from build123d import *

# Parameters (mm, degrees)
SKETCH1_R           = 24
SKETCH1_R_2         = 2
SKETCH1_R_3         = 1.5
BOSS_EXTRUDE1_DEPTH = 2
CUT_EXTRUDE1_DEPTH  = 2
FILLET1_R           = 1.5
SKETCH3_R           = 1.75
CUT_EXTRUDE2_DEPTH  = 10
SCALE1_SCALE        = 2
SKETCH4_R           = 5
CUT_EXTRUDE3_DEPTH  = 10
SKETCH5_R           = 6.547213639
SKETCH5_R_2         = 2.5
SKETCH5_R_3         = 5.064875416
BOSS_EXTRUDE2_DEPTH = 4


with BuildPart() as part:
    # Sketch1 → Boss-Extrude1 (new body)
    with BuildSketch(Plane(origin=(0, 0, 0), x_dir=(1, 0, 0), z_dir=(0, 1, 0))):
        with Locations(Location((0, 0, 0), (0, 0, 270))):
            Circle(SKETCH1_R)
        with Locations(Location((0, 0, 0), (0, 0, 270))):
            Circle(SKETCH1_R_2, mode=Mode.SUBTRACT)
        with Locations(Location((11.5, 0, 0), (0, 0, 270))):
            Circle(SKETCH1_R_3, mode=Mode.SUBTRACT)
        with Locations(Location((-5.75, -9.959292144, 0), (0, 0, 270))):
            Circle(SKETCH1_R_3, mode=Mode.SUBTRACT)
        with Locations(Location((-5.75, 9.959292144, 0), (0, 0, 270))):
            Circle(SKETCH1_R_3, mode=Mode.SUBTRACT)
    extrude(amount=BOSS_EXTRUDE1_DEPTH)

    # Sketch2 → Cut-Extrude1 (cut)
    with BuildSketch(Plane(origin=(0, 2, 0), x_dir=(1, 0, 0), z_dir=(0, 1, 0))):
        with BuildLine():
            Line((21.972994789, 3.5), (14.585952146, 3.5))
            ThreePointArc((14.585952146, 3.5), (7.5, 12.990381057), (-4.26188716, 14.381805097))
            Line((-4.26188716, 14.381805097), (-7.955408481, 20.779171685))
            ThreePointArc((-7.955408481, 20.779171685), (11.125, 19.269065234), (21.972994789, 3.5))
        make_face()
        with BuildLine():
            Line((21.972994789, -3.5), (14.585952146, -3.5))
            ThreePointArc((14.585952146, -3.5), (7.5, -12.990381057), (-4.26188716, -14.381805097))
            Line((-4.26188716, -14.381805097), (-7.955408481, -20.779171685))
            ThreePointArc((-7.955408481, -20.779171685), (11.125, -19.269065234), (21.972994789, -3.5))
        make_face()
        with BuildLine():
            Line((-14.017586308, -17.279171685), (-10.324064986, -10.881805097))
            ThreePointArc((-10.324064986, -10.881805097), (-15, 0), (-10.324064986, 10.881805097))
            Line((-10.324064986, 10.881805097), (-14.017586308, 17.279171685))
            ThreePointArc((-14.017586308, 17.279171685), (-22.25, 0), (-14.017586308, -17.279171685))
        make_face()
    extrude(amount=-CUT_EXTRUDE1_DEPTH, mode=Mode.SUBTRACT)

    # Fillet1
    fillet1_edges = [part.edges().sort_by_distance(p)[0] for p in [
        (-7.955408481, 1, -20.779171685),
        (21.972994789, 1, -3.5),
        (14.585952146, 1, -3.5),
        (-4.26188716, 1, -14.381805097),
        (-14.017586308, 1, 17.279171685),
        (-14.017586308, 1, -17.279171685),
        (-10.324064986, 1, -10.881805097),
        (-10.324064986, 1, 10.881805097),
        (21.972994789, 1, 3.5),
        (-7.955408481, 1, 20.779171685),
        (-4.26188716, 1, 14.381805097),
        (14.585952146, 1, 3.5),
    ]]
    fillet(fillet1_edges, radius=FILLET1_R)

    # Sketch3 → Cut-Extrude2 (cut)
    with BuildSketch(Plane(origin=(0, 2, 0), x_dir=(1, 0, 0), z_dir=(0, 1, 0))):
        with Locations(Location((5, 8.660254038, 0), (0, 0, 270))):
            Circle(SKETCH3_R)
        with Locations(Location((5, -8.660254038, 0), (0, 0, 270))):
            Circle(SKETCH3_R)
        with Locations(Location((-10, 0, 0), (0, 0, 270))):
            Circle(SKETCH3_R)
    extrude(amount=-CUT_EXTRUDE2_DEPTH, mode=Mode.SUBTRACT)


with BuildPart() as part_1:
    # Scale1: scaled about (0, 1, 0)
    add(part.part.scale(SCALE1_SCALE).moved(Location((0, -1, 0))))

    # Sketch4 → Cut-Extrude3 (cut)
    with BuildSketch(Plane(origin=(0, 3, 0), x_dir=(1, 0, 0), z_dir=(0, 1, 0))):
        with Locations(Location((0, 0, 0), (0, 0, 270))):
            Circle(SKETCH4_R)
    extrude(amount=-CUT_EXTRUDE3_DEPTH, mode=Mode.SUBTRACT)

    # Sketch5 → Boss-Extrude2 (add)
    # profile 1 of 6: a face of its own
    with BuildSketch(Plane(origin=(0, 3, 0), x_dir=(1, 0, 0), z_dir=(0, 1, 0))):
        with Locations((10, 17.320508076)):
            Circle(SKETCH5_R)
        with Locations(Location((10, 17.320508076, 0), (0, 0, 270))):
            Circle(SKETCH5_R_2, mode=Mode.SUBTRACT)
    # profile 2 of 6: a face of its own
    with BuildSketch(Plane(origin=(0, 3, 0), x_dir=(1, 0, 0), z_dir=(0, 1, 0))):
        with Locations((10, -17.320508076)):
            Circle(SKETCH5_R)
        with Locations(Location((10, -17.320508076, 0), (0, 0, 270))):
            Circle(SKETCH5_R_2, mode=Mode.SUBTRACT)
    # profile 3 of 6: a face of its own
    with BuildSketch(Plane(origin=(0, 3, 0), x_dir=(1, 0, 0), z_dir=(0, 1, 0))):
        with Locations((-20, 0)):
            Circle(SKETCH5_R)
        with Locations(Location((-20, 0, 0), (0, 0, 270))):
            Circle(SKETCH5_R_2, mode=Mode.SUBTRACT)
    # profile 4 of 6: a face of its own
    with BuildSketch(Plane(origin=(0, 3, 0), x_dir=(1, 0, 0), z_dir=(0, 1, 0))):
        with Locations((-11.5, 19.918584287)):
            Circle(SKETCH5_R_3)
        with Locations(Location((-11.5, 19.918584287, 0), (0, 0, 270))):
            Circle(SKETCH5_R_2, mode=Mode.SUBTRACT)
    # profile 5 of 6: a face of its own
    with BuildSketch(Plane(origin=(0, 3, 0), x_dir=(1, 0, 0), z_dir=(0, 1, 0))):
        with Locations((23, 0)):
            Circle(SKETCH5_R_3)
        with Locations(Location((23, 0, 0), (0, 0, 270))):
            Circle(SKETCH5_R_2, mode=Mode.SUBTRACT)
    # profile 6 of 6: a face of its own
    with BuildSketch(Plane(origin=(0, 3, 0), x_dir=(1, 0, 0), z_dir=(0, 1, 0))):
        with Locations((-11.5, -19.918584287)):
            Circle(SKETCH5_R_3)
        with Locations(Location((-11.5, -19.918584287, 0), (0, 0, 270))):
            Circle(SKETCH5_R_2, mode=Mode.SUBTRACT)
    extrude(amount=-BOSS_EXTRUDE2_DEPTH)


solid = part_1.part
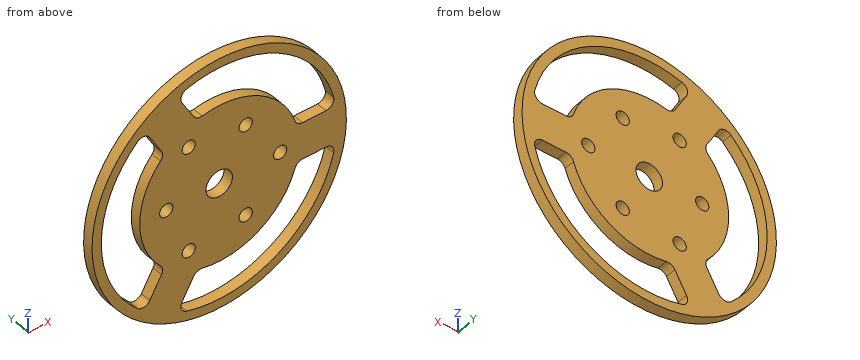
Build history of the part. All positions in model axes, mm. Coordinates: 2 decimals unless noted, no trailing zeros. Order: outer loops, then holes, each group sorted by start corner. A loop starts at its lowest first (then second) coordinate and runs counter-clockwise, first axis right, second up. Notation, with made-up numbers: (67, -7) - (75, -7) arc R17 ccw to (75, 1) - close; hole circle Ø1 at (72, -11.5). An arc over 180 degrees is marked (long way). Put each result on its own line as item: value.
1. Saw through at D-D (y = 1.1). Give the number of separate pieces and of enclosed holes in the cut face, and give its area (3 significant figures).
Answer sheet:
separate pieces: 1
enclosed holes: 10
area: 4,290 mm^2
2. Saw through at B-B (x = 0). Write the cut outline in (y, z), and give its area (3 significant figures).
Answer sheet:
outline: (-1, -48) - (3, -48) - (3, -44.5) - (-1, -44.5) - close; (-1, -30) - (3, -30) - (3, -5) - (-1, -5) - close; (-1, 5) - (3, 5) - (3, 30) - (-1, 30) - close; (-1, 44.5) - (3, 44.5) - (3, 48) - (-1, 48) - close
area: 228 mm^2
3. Probe line 1 along Z through (x, y) = (36, 0.35); line 2 along X through (y, z) = (0.25, 4); line 3 along Z through (x, y) = (38, -0.05). List the from-to ranges inside material, lowest first. Write a range as [from, to].
Answer sheet:
line 1: z = [-31.75, -26.16], [-7, 7], [26.16, 31.75]
line 2: x = [-47.83, -44.32], [-29.73, -3], [3, 47.83]
line 3: z = [-29.33, -23.16], [-7, 7], [23.16, 29.33]
4. Drop flat-ended pins along their axis: P1, Ø9, axis at x = 0, z = 0, coming from the -Y side; P2, Ø2, axis at y = 0, z = 25.5, coming from the -X side; P3, Ø2, axis at x = 36, y = 0.5, coming from the +Z side; P4, Ø1.5, axis at x = 20, y = 0.5, coming from the -Z side. Give the stop position or say it passes through.
Answer sheet:
P1: passes through
P2: stops at x = -41.28
P3: stops at z = 32.85
P4: stops at z = -43.97
5. Saw through at C-C (x = -20). Write the cut outline in (y, z), and give its area (3 significant figures).
Answer sheet:
outline: (-1, -43.63) - (3, -43.63) - (3, -2.5) - (-1, -2.5) - close; (-1, 2.5) - (3, 2.5) - (3, 43.63) - (-1, 43.63) - close
area: 329 mm^2
6. Saw through at A-A (z = 0). Write the cut outline in (x, y), and give its area (3 significant figures).
Answer sheet:
outline: (-48, -1) - (-44.5, -1) - (-44.5, 3) - (-48, 3) - close; (-30, -1) - (-22.5, -1) - (-22.5, 3) - (-30, 3) - close; (-17.5, -1) - (-5, -1) - (-5, 3) - (-17.5, 3) - close; (5, -1) - (20.5, -1) - (20.5, 3) - (5, 3) - close; (25.5, -1) - (48, -1) - (48, 3) - (25.5, 3) - close
area: 246 mm^2
